Check sheet for the modelled part. Datum: model origin and axes. Units: mm. A direction names the side the tool comes from. Coordinates: 2 decimals unless noted, no trailing zeros. Write each loop counter-clockwise with the first axis right and the second up, starting at its lowest first coordinate (ties: lowest second). Pieces come first, ordered by that corner, then holes. Notation, with made-up numbers: (53.25, 67.25) -> (91.25, 67.25) arc R7 ccw to (91.25, 73.25) -> close; hole circle Ø11 at (72.5, 85). An arc over 180 degrees is marked (long way). One line per item, written item: value. Start each with the question number.
1) Sectioned sample at A-A on z = 1.8. Enter the section's corners in (x, y).
2) Sectioned sample at B-B on y = 6.5. Enter the section's corners in (x, z).
3) Set-up check for faces 5 (the flat face through (14.428, 3.477, 0.493)), 6 (the flat face through (16, 4, 3)): record each of +Z, -Z, +X, -X, +Y, -Y from which the full face is reachable in a straight line by a thin tool's end or side.
4) Draft check along Y on faces 1 (the cylindrical face through (54.336, 3.368, 1.479)), 2 (the flat face through (16, 0, 1)), 3 (the flat face through (14.85, 3.33, 0.49)), 4 (the flat face through (15, 7.999, 1)). Enter one of: +Y half, -Y half, draft (parallel to the pull), parting line (faces both ways), or undercut.
5) Scan lines: line 1 along X through (y, z) = (3.75, 2.5); line 2 along X through (y, z) = (4.75, 1.65); line 3 along Y through (x, z) = (-24, 0.8). Record each from-to range of solid material in increasing order. Write a range as [from, to].
6) Gauge pin test, flat end, axial feed: P1, Ø1, axis at y = 2.5, z = 2, coming from the +X side. Record the tip position at first contact, or that the pin passes through.
```python
from build123d import *

# Parameters (mm, degrees)
SKETCH_1_R          = 1.65
EXTRUDE_1_DEPTH     = 3
CUT_EXTRUDE_1_DEPTH = 1


with BuildPart() as part:
    # 草图1 → 凸台-拉伸1 (new body)
    with BuildSketch(Plane(origin=(0, 0, 0), x_dir=(-1, 0, 0), z_dir=(0, 0, -1))):
        with BuildLine():
            Line((-55.860221974, 0), (24.13832066, 0))
            ThreePointArc((24.13832066, 0), (26.966394209, 1.171219344), (28.138320535, 3.999))
            ThreePointArc((28.138320535, 3.999), (26.96674766, 6.827427125), (24.138320535, 7.999))
            Line((24.138320535, 7.999), (-55.860222099, 7.999))
            ThreePointArc((-55.860222099, 7.999), (-58.688295648, 6.827780656), (-59.860221974, 4))
            ThreePointArc((-59.860221974, 4), (-58.688649099, 1.171572875), (-55.860221974, 0))
        make_face()
        with Locations((24.138809001, 3.998511534)):
            Circle(SKETCH_1_R, mode=Mode.SUBTRACT)
        with Locations((-55.859733508, 3.999511534)):
            Circle(SKETCH_1_R, mode=Mode.SUBTRACT)
    extrude(amount=-EXTRUDE_1_DEPTH)

    # 草图2 → 切除-拉伸1 (cut)
    with BuildSketch(Plane(origin=(0, 0, 0), x_dir=(-1, 0, 0), z_dir=(0, 0, -1))):
        Polygon((-15.675290893, 5.246411073), (-13.52144474, 5.246411073), (-15.361188329, 1.656667483), (-15.632522464, 1.806006425), (-14.05289506, 4.887436714), (-15.675290893, 4.887436714), align=None)
    extrude(amount=-CUT_EXTRUDE_1_DEPTH, mode=Mode.SUBTRACT)


solid = part.part
```
Answers:
1. outline: (-28.14, 4) arc R4 ccw to (-24.14, 0) -> (55.86, 0) arc R4 ccw to (59.86, 4) arc R4 ccw to (55.86, 8) -> (-24.14, 8) arc R4 ccw to start; hole circle Ø3.3 at (-24.14, 4); hole circle Ø3.3 at (55.86, 4)
2. outline: (-27.26, 0) -> (58.98, 0) -> (58.98, 3) -> (-27.26, 3) -> close
3. face 5: -Z
3. face 6: +Z, +X, -X, +Y, -Y
4. face 1: undercut
4. face 2: -Y half
4. face 3: undercut
4. face 4: +Y half
5. line 1: x = [-28.13, -25.77], [-22.51, 54.23], [57.49, 59.85]
5. line 2: x = [-28.07, -25.61], [-22.67, 54.39], [57.33, 59.79]
5. line 3: y = [0, 2.35], [5.64, 8]
6. P1: stops at x = 59.73
